Part model, mm, in its own coordinate system. Face numbers are marked on the shaded views. A direction names the side the tool comes from. Round coordinates to 2 decimals unless told otherwise and drop trailing zeros. Write each loop counter-clockwise with the first axis right and the second up, starting at its lowest first coordinate (ties: lowest second). Pieces come first, ordered by that corner, then holes. Notation, with made-up numbers: (-5.75, 30) -> (26.25, 30) arc R11 cw to (26.25, 41) -> close; hole circle Ø11 at (24.5, 12.5). An arc over 180 degrees is marked (long way). Use CSV: the item, a comma, the result in double quotes. Start each with the question number.
(1) Saw through at A-A (y = -3). Give the cut face in (x, z), plus the area to 3 significant figures.
(2) Probe line 1 (Y direction, x = 1, z = 0); line 2 (Y direction, x = -2.5, z = -1); line 3 (X direction, y = -21, z = -4). List the from-to ranges inside material, lowest first. Write a range as [from, to].
(3) Saw through at B-B (y = -32). Give the cut face in (x, z), plus the area to 3 significant figures.
(4) Which spindle directions (+Z, -Z, +X, -X, +Y, -Y) get a long thin tool onto all of the face, cutting with end or side? Do the marked faces 1, 2 and 3. Say none if no direction does.
(5) Drop flat-ended pins along their axis: pin 1 (3 mm diameter, centred on x = -0.5, y = -7.5, fed in from +Z); pin 2 (5 mm diameter, centred on x = -7, y = -22, fed in from +Z); pin 3 (4 mm diameter, centred on x = 1, y = -9, fed in from -Z). Give the stop position or say it passes through.
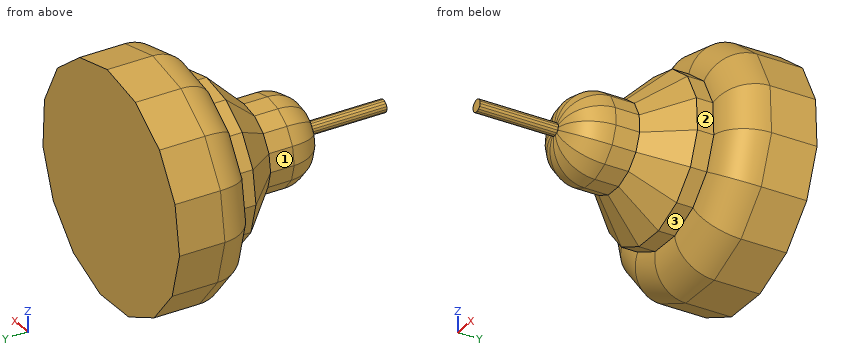
```python
from build123d import *

# Parameters (mm, degrees)
F1_DEPTH = 11.43
F2_R     = 5.08
F3_DEPTH = 2.286
F4_DEPTH = 5.08
F5_SIZE  = 5.08
F6_DEPTH = 8.382
F7_R     = 5.08
F8_DEPTH = 10.922


with BuildPart() as f1:
    # F0 (on Front) → F1 (new body)
    with BuildSketch(Plane.XZ):
        Polygon((-5.8849686034, 15.3612454542), (-11.6241677455, 11.6395636341), (-15.3534426822, 5.9052955195), (-16.4279678975, -0.8500518383), (-14.6619482199, -7.4584175109), (-10.3607444954, -12.7771550382), (-4.2680739233, -15.8866063825), (2.5625854044, -16.2491191581), (8.9501504353, -13.8020116126), (13.7901531464, -8.968410872), (16.2457130989, -2.5840904161), (15.8922416689, 4.2470427484), (12.7908572779, 10.3438236386), (7.4778174622, 14.652063451), (0.8717950735, 16.4268283828), align=None)
    extrude(amount=F1_DEPTH)

    # F2
    f2_edges = [f1.edges().sort_by_distance(p)[0] for p in [
        (-2.506587, -11.43, 15.894037),
        (-8.754568, -11.43, 13.500405),
        (-13.488805, -11.43, 8.77243),
        (-15.890705, -11.43, 2.527622),
        (-15.544958, -11.43, -4.154235),
        (-12.511346, -11.43, -10.117786),
        (-7.314409, -11.43, -14.331881),
        (-0.852744, -11.43, -16.067863),
        (5.756368, -11.43, -15.025565),
        (11.370152, -11.43, -11.385211),
        (15.017933, -11.43, -5.776251),
        (16.068977, -11.43, 0.831476),
        (14.341549, -11.43, 7.295433),
        (10.134337, -11.43, 12.497944),
        (4.174806, -11.43, 15.539446),
    ]]
    fillet(f2_edges, radius=F2_R)

    # F3 (add): a face of the model
    f3_faces = [f1.faces().sort_by_distance(p)[0] for p in [
        (0, -11.43, 0),
    ]]
    extrude(f3_faces, amount=F3_DEPTH)

    # F4 (add): a face of the model
    f4_faces = [f1.faces().sort_by_distance(p)[0] for p in [
        (0, -13.716, 0),
    ]]
    extrude(f4_faces, amount=F4_DEPTH)

    # F5
    f5_edges = [f1.edges().sort_by_distance(p)[0] for p in [
        (-5.990622, -18.796, 9.238128),
        (-1.71522, -18.796, 10.876055),
        (2.856758, -18.796, 10.633414),
        (6.934778, -18.796, 8.552159),
        (9.813711, -18.796, 4.992157),
        (10.995765, -18.796, 0.568967),
        (10.27655, -18.796, -3.952603),
        (7.780427, -18.796, -7.790732),
        (3.938998, -18.796, -10.281773),
        (-0.58352, -18.796, -10.995002),
        (-5.005142, -18.796, -9.807095),
        (-8.56133, -18.796, -6.923452),
        (-10.637186, -18.796, -2.842682),
        (-10.873776, -18.796, 1.729614),
        (-9.230191, -18.796, 6.002844),
    ]]
    chamfer(f5_edges, length=F5_SIZE)

    # F6 (add): a face of the model
    f6_faces = [f1.faces().sort_by_distance(p)[0] for p in [
        (0, -18.796, 0),
    ]]
    extrude(f6_faces, amount=F6_DEPTH)

    # F7
    f7_edges = [f1.edges().sort_by_distance(p)[0] for p in [
        (-3.226676, -27.178, 4.975851),
        (-0.923854, -27.178, 5.858074),
        (-4.971576, -27.178, 3.233259),
        (1.538711, -27.178, 5.727382),
        (-5.856846, -27.178, 0.931607),
        (3.735218, -27.178, 4.606374),
        (-5.729414, -27.178, -1.531129),
        (5.285873, -27.178, 2.688882),
        (-4.611314, -27.178, -3.729118),
        (5.922552, -27.178, 0.306458),
        (-2.695876, -27.178, -5.282309),
        (5.535168, -27.178, -2.128956),
        (-0.314296, -27.178, -5.922141),
        (4.190703, -27.178, -4.196253),
        (2.121628, -27.178, -5.537981),
    ]]
    fillet(f7_edges, radius=F7_R)

    # F8 (add): a face of the model
    f8_faces = [f1.faces().sort_by_distance(p)[0] for p in [
        (0, -27.178, 0),
    ]]
    extrude(f8_faces, amount=F8_DEPTH)


solid = f1.part
```
Answers:
1,outline,"(-16.43, -0.85) -> (-14.66, -7.46) -> (-10.36, -12.78) -> (-4.27, -15.89) -> (2.56, -16.25) -> (8.95, -13.8) -> (13.79, -8.97) -> (16.25, -2.58) -> (15.89, 4.25) -> (12.79, 10.34) -> (7.48, 14.65) -> (0.87, 16.43) -> (-5.88, 15.36) -> (-11.62, 11.64) -> (-15.35, 5.91) -> close"
1,area,"825 mm²"
2,line 1,"y = [-27.18, 0]"
2,line 2,"y = [-26.84, 0]"
2,line 3,"x = [-4.39, 4.39]"
3,outline,"(-0.87, -0.04) -> (-0.77, -0.39) -> (-0.55, -0.68) -> (-0.23, -0.84) -> (0.14, -0.86) -> (0.47, -0.73) -> (0.73, -0.47) -> (0.86, -0.14) -> (0.84, 0.22) -> (0.68, 0.55) -> (0.4, 0.77) -> (0.05, 0.87) -> (-0.31, 0.81) -> (-0.61, 0.62) -> (-0.81, 0.31) -> close"
3,area,"2.31 mm²"
4,face 1,"+Z, -X, -Y"
4,face 2,"+Z, +X, -Y"
4,face 3,"-Z, +X, -Y"
5,pin 1,"stops at z = 16.4"
5,pin 2,"stops at z = 3.96"
5,pin 3,"stops at z = -16.14"
